Input: part model. Units: mm. Frame: model coordinates. Face numbers are marked on the shaded views. A direction names the side the tool comes from. Round coordinates to 2 decimals unless told otherwise and drop trailing zeros. Write each loop counter-clockwise with the first axis right and the second up, starting at its lowest first coordinate (ties: lowest second). Pieces come first, ordered by that corner, then holes. Notation, with made-up numbers: (-3.5, 15.25) -> (38.5, 15.25) arc R26 ccw to (38.5, 36.25) -> close; hole circle Ø8 at (-1.75, 69). An arc over 180 degrees is marked (long way). Write item = value, one per line.
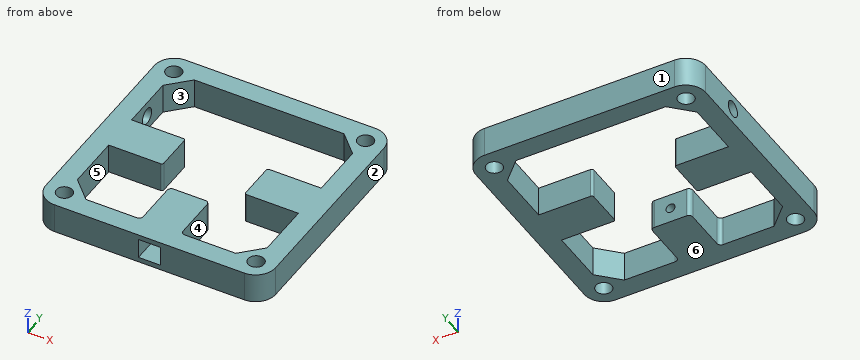
```python
from build123d import *

# Parameters (mm, degrees)
SKETCH1_W           = 115
SKETCH1_H           = 115
SKETCH1_W_2         = 95
SKETCH1_H_2         = 95
BOSS_EXTRUDE1_DEPTH = 15
SKETCH10_W          = 20
SKETCH10_H          = 15
BOSS_EXTRUDE4_DEPTH = 27
SKETCH3_W           = 11
SKETCH3_H           = 10
CUT_EXTRUDE1_DEPTH  = 28
FILLET1_R           = 10
CHAMFER1_SIZE       = 10
SKETCH4_R           = 4
CUT_EXTRUDE3_DEPTH  = 57.5
SKETCH9_R           = 4
CUT_EXTRUDE7_DEPTH  = 30
FILLET6_R           = 2
SKETCH11_R          = 2.25
CUT_EXTRUDE8_DEPTH  = 30
SKETCH12_W          = 95
SKETCH12_H          = 20
BOSS_EXTRUDE5_DEPTH = 15
SKETCH13_W          = 41
SKETCH13_H          = 27.815570672
CUT_EXTRUDE9_DEPTH  = 20
FILLET7_R           = 1


with BuildPart() as part:
    # Sketch1 → Boss-Extrude1 (new body)
    with BuildSketch(Plane.XY.offset(-13)):
        Rectangle(SKETCH1_W, SKETCH1_H)
        Rectangle(SKETCH1_W_2, SKETCH1_H_2, mode=Mode.SUBTRACT)
    extrude(amount=BOSS_EXTRUDE1_DEPTH)

    # Sketch10 → Boss-Extrude4 (add)
    with BuildSketch(Plane(origin=(0, -22.4, 0), x_dir=(1, 0, 0), z_dir=(0, 1, 0))):
        with Locations((0, 5.5)):
            Rectangle(SKETCH10_W, SKETCH10_H)
    extrude(amount=-BOSS_EXTRUDE4_DEPTH)

    # Sketch3 → Cut-Extrude1 (cut)
    with BuildSketch(Plane(origin=(0, -57.5, 0), x_dir=(-1, 0, 0), z_dir=(0, -1, 0))):
        with Locations((0, 5.5)):
            Rectangle(SKETCH3_W, SKETCH3_H)
    extrude(amount=-CUT_EXTRUDE1_DEPTH, mode=Mode.SUBTRACT)

    # Fillet1
    fillet1_edges = [part.edges().sort_by_distance(p)[0] for p in [
        (-57.5, 57.5, -5.5),
        (57.5, 57.5, -5.5),
        (57.5, -57.5, -5.5),
        (-57.5, -57.5, -5.5),
    ]]
    fillet(fillet1_edges, radius=FILLET1_R)

    # Chamfer1
    chamfer1_edges = [part.edges().sort_by_distance(p)[0] for p in [
        (-47.5, 47.5, -5.5),
        (-47.5, -47.5, -5.5),
        (47.5, -47.5, -5.5),
        (47.5, 47.5, -5.5),
    ]]
    chamfer(chamfer1_edges, length=CHAMFER1_SIZE)

    # Sketch4 → Cut-Extrude3 (cut, symmetric)
    with BuildSketch(Plane.XY):
        with Locations(Location((-48, 48, 0), (0, 0, 180))):
            Circle(SKETCH4_R)
        with Locations(Location((48, 48, 0), (0, 0, 180))):
            Circle(SKETCH4_R)
        with Locations(Location((48, -48, 0), (0, 0, 180))):
            Circle(SKETCH4_R)
        with Locations(Location((-48, -48, 0), (0, 0, 180))):
            Circle(SKETCH4_R)
    extrude(amount=CUT_EXTRUDE3_DEPTH, both=True, mode=Mode.SUBTRACT)

    # Sketch9 → Cut-Extrude7 (cut)
    with BuildSketch(Plane.ZY.offset(57.5)):
        with Locations(Location((-5.5, 23.6, 0), (0, 0, 270))):
            Circle(SKETCH9_R)
    extrude(amount=-CUT_EXTRUDE7_DEPTH, mode=Mode.SUBTRACT)

    # Fillet6
    fillet6_edges = [part.edges().sort_by_distance(p)[0] for p in [
        (10, -47.5, -5.5),
        (-10, -47.5, -5.5),
        (-10, -22.4, -5.5),
        (10, -22.4, -5.5),
    ]]
    fillet(fillet6_edges, radius=FILLET6_R)

    # Sketch11 → Cut-Extrude8 (cut)
    with BuildSketch(Plane(origin=(0, -29.5, 0), x_dir=(-1, 0, 0), z_dir=(0, -1, 0))):
        with Locations(Location((0, 5.5, 0), (0, 0, 90))):
            Circle(SKETCH11_R)
    extrude(amount=-CUT_EXTRUDE8_DEPTH, mode=Mode.SUBTRACT)

    # Sketch12 → Boss-Extrude5 (add)
    with BuildSketch(Plane.XY.offset(2)):
        Rectangle(SKETCH12_W, SKETCH12_H)
    extrude(amount=-BOSS_EXTRUDE5_DEPTH)

    # Sketch13 → Cut-Extrude9 (cut)
    with BuildSketch(Plane.XY.offset(2)):
        Rectangle(SKETCH13_W, SKETCH13_H)
    extrude(amount=-CUT_EXTRUDE9_DEPTH, mode=Mode.SUBTRACT)

    # Fillet7
    fillet7_edges = [part.edges().sort_by_distance(p)[0] for p in [
        (-20.5, -10, -5.5),
        (20.5, -10, -5.5),
        (20.5, 10, -5.5),
        (-20.5, 10, -5.5),
    ]]
    fillet(fillet7_edges, radius=FILLET7_R)


solid = part.part
```
1) Cut plane C-C (z = -5.5). Count the separate pieces of the cut face and the enclosed holes in it, and give its area (3 significant figures).
Solutions:
separate_pieces = 2
enclosed_holes = 4
area = 5,270 mm^2
2) Cut plane D-D (x = 0). Return the cut outline in (y, z).
Solutions:
outline = (-57.5, -13) -> (-22.4, -13) -> (-22.4, -7.75) -> (-29.5, -7.75) -> (-29.5, -10.5) -> (-57.5, -10.5) -> close; (-57.5, -0.5) -> (-29.5, -0.5) -> (-29.5, -3.25) -> (-22.4, -3.25) -> (-22.4, 2) -> (-57.5, 2) -> close; (47.5, -13) -> (57.5, -13) -> (57.5, 2) -> (47.5, 2) -> close
3) Cut plane A-A (x = 28). Return the cut outline in (y, z).
Solutions:
outline = (-57.5, -13) -> (-47.5, -13) -> (-47.5, 2) -> (-57.5, 2) -> close; (-10, -13) -> (10, -13) -> (10, 2) -> (-10, 2) -> close; (47.5, -13) -> (57.5, -13) -> (57.5, 2) -> (47.5, 2) -> close
4) Access query for the marked faces 5 and 6. Directions: +Z, -Z, +X, -X, +Y, -Y. A direction counts if a zero-diameter tool reaches every point of the face in a straight line with its end or side. Return the directions, or none.
Solutions:
face_5 = +Z, -Z
face_6 = -Z, +X, -X, +Y, -Y
5) Line query: L1, parallel to X at y = -48, z = -2.25; L2, parallel to Y at x = -30.5, z = -5.5; L3, parallel to Y at x = -48, z = -6. Output: solid intervals per line, ascending. Write a range as from..to.
Solutions:
L1 = -57.49..-52, -44..-5.5, 5.5..44, 52..57.49
L2 = -57.5..-47.5, -10..10, 47.5..57.5
L3 = -57.49..-52, -44..19.63, 27.57..44, 52..57.49
6) Draft query along X for the marked faces 1, 2, 3 and 4. Return one class per face: +X half, -X half, draft (parallel to the pull), parting line (faces both ways), or undercut.
Solutions:
face_1 = draft
face_2 = +X half
face_3 = undercut
face_4 = undercut
7) Cut plane B-B (y = 23.6). Return the cut outline in (x, z).
Solutions:
outline = (-57.5, -13) -> (-47.5, -13) -> (-47.5, -9.5) -> (-57.5, -9.5) -> close; (-57.5, -1.5) -> (-47.5, -1.5) -> (-47.5, 2) -> (-57.5, 2) -> close; (47.5, -13) -> (57.5, -13) -> (57.5, 2) -> (47.5, 2) -> close
8) First-contact query: P1, Ø12, axis at x = -13.5, y = 43, coming from the -Z side; P2, Ø5, axis at x = 2, z = -5, coming from the -Y side. Flat tips, straight axial feed; report the tip coordinate or a pass-through.
Solutions:
P1 = -13
P2 = -29.5
